Read the model definition and answer for the solid it produces. Units are mm, in the model's axes. Face numbers are marked on the shaded views. A direction names the side the tool comes from. Round coordinates to 2 decimals unless told otherwise and drop trailing zeros. Order: outer loops, then holes, each group sorted by start corner. A loop starts at its lowest first (then second) coordinate and runs counter-clockwise, first axis right, second up. Notation, with made-up numbers: (60.5, 45.5) - (104.5, 45.5) arc R19 ccw to (104.5, 69.5) - close; hole circle Ø4 at (-40, 4). An arc over 180 degrees is marked (long way). Answer as a JSON object with one key per item and string values. Group by question number.
Q1. A cutting plane is placed at A-A on x = 0.5. Determine the outline of the cut face in (y, z).
Q2. Given pin 1 Ø0.5 at (x, z) = (3.5, 0) entering from +Y; pin 2 Ø0.7 at (y, z) = (0, 2) entering from +X, each flat-ended and moving along its own axis, determine where each tip first touches the part or whether it passes through.
Q3. A cutting plane is placed at B-B on y = 0.55. Determine the outline of the cut face in (x, z) (3 decimals), and give its area (3 significant figures).
Q4. A tool of negligible diameter and unlimited length cuts with its end or side. For the marked faces 1 and 2, from which of +Z, -Z, +X, -X, +Y, -Y can it reach the whole face along a straight path? Write none if from no direction.
Q5. Consider line 1 (X direction, y = 0.55, z = 1); line 2 (Z direction, x = -1.5, y = 0.25); line 3 (X direction, y = -0.45, z = 2) (3 decimals). Determine where each line is inside the solid, lowest interval first.
Q6. A cutting plane is placed at D-D on y = -0.8. Determine the outline of the cut face in (x, z), and give its area (3 significant figures).
Q7. A cutting plane is placed at C-C on z = 1.1. Determine the outline of the cut face in (x, y), and give its area (3 significant figures).
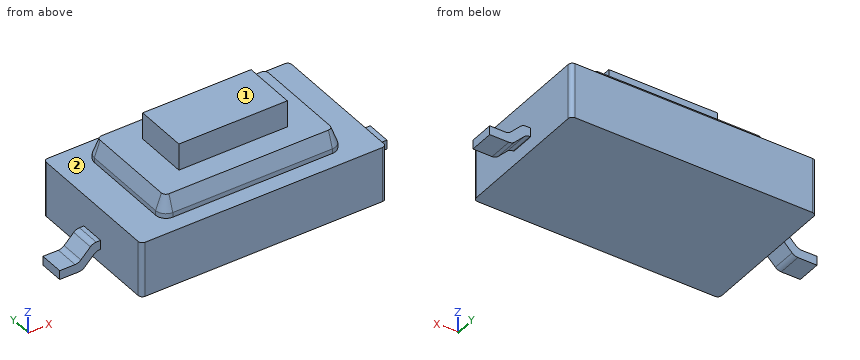
```python
from build123d import *

# Parameters (mm, degrees)
BOSS_EXTRUDE1_DEPTH = 1.35
BOSS_EXTRUDE2_DEPTH = 1.85
SKETCH1_4_W         = 2.65
SKETCH1_4_H         = 1.3
BOSS_EXTRUDE3_DEPTH = 2.5
CHAMFER1_SIZE       = 0.14
CHAMFER1_SIZE2      = 0.384646839
BOSS_EXTRUDE4_DEPTH = 0.3


with BuildPart() as part:
    # Sketch1 → Boss-Extrude1 (new body)
    with BuildSketch(Plane.XY):
        with BuildLine():
            Line((-2.9, 1.75), (2.9, 1.75))
            ThreePointArc((2.9, 1.75), (2.970710678, 1.720710678), (3, 1.65))
            Line((3, 1.65), (3, -1.65))
            ThreePointArc((3, -1.65), (2.970710678, -1.720710678), (2.9, -1.75))
            Line((2.9, -1.75), (-2.9, -1.75))
            ThreePointArc((-2.9, -1.75), (-2.970710678, -1.720710678), (-3, -1.65))
            Line((-3, -1.65), (-3, 1.65))
            ThreePointArc((-3, 1.65), (-2.970710678, 1.720710678), (-2.9, 1.75))
        make_face()
    extrude(amount=BOSS_EXTRUDE1_DEPTH)

    # Sketch1<3> → Boss-Extrude2 (add)
    with BuildSketch(Plane.XY):
        with BuildLine():
            Line((-1.95, 1.35), (1.95, 1.35))
            ThreePointArc((1.95, 1.35), (2.126776695, 1.276776695), (2.2, 1.1))
            Line((2.2, 1.1), (2.2, -1.1))
            ThreePointArc((2.2, -1.1), (2.126776695, -1.276776695), (1.95, -1.35))
            Line((1.95, -1.35), (-1.95, -1.35))
            ThreePointArc((-1.95, -1.35), (-2.126776695, -1.276776695), (-2.2, -1.1))
            Line((-2.2, -1.1), (-2.2, 1.1))
            ThreePointArc((-2.2, 1.1), (-2.126776695, 1.276776695), (-1.95, 1.35))
        make_face()
    extrude(amount=BOSS_EXTRUDE2_DEPTH)

    # Sketch1<4> → Boss-Extrude3 (add)
    with BuildSketch(Plane.XY):
        Rectangle(SKETCH1_4_W, SKETCH1_4_H)
    extrude(amount=BOSS_EXTRUDE3_DEPTH)

    # Chamfer1
    chamfer1_edges = [part.edges().sort_by_distance(p)[0] for p in [
        (0, -1.35, 1.85),
        (-2.126776695, -1.276776695, 1.85),
        (-2.2, 0, 1.85),
        (-2.126776695, 1.276776695, 1.85),
        (2.2, 0, 1.85),
        (2.126776695, 1.276776695, 1.85),
        (0, 1.35, 1.85),
    ]]
    chamfer1_side = [part.faces().sort_by_distance(p)[0] for p in [
        (0, 1.298376362, 1.85),
    ]]
    chamfer(chamfer1_edges, length=CHAMFER1_SIZE, length2=CHAMFER1_SIZE2, reference=chamfer1_side[0])

    # Sketch2 → Boss-Extrude4 (add, symmetric)
    with BuildSketch(Plane(origin=(0, 0, 0), x_dir=(1, 0, 0), z_dir=(0, 1, 0))):
        with BuildLine():
            Line((3, -0.35), (3.017157288, -0.35))
            ThreePointArc((3.017157288, -0.35), (3.093693974, -0.334775907), (3.158578644, -0.291421356))
            Line((3.158578644, -0.291421356), (3.391421356, -0.058578644))
            ThreePointArc((3.391421356, -0.058578644), (3.456306026, -0.015224093), (3.532842712, 0))
            Line((3.532842712, 0), (4, 0))
            Line((4, 0), (4, -0.22))
            Line((4, -0.22), (3.623969696, -0.22))
            ThreePointArc((3.623969696, -0.22), (3.54743301, -0.235224093), (3.48254834, -0.278578644))
            Line((3.48254834, -0.278578644), (3.249705627, -0.511421356))
            ThreePointArc((3.249705627, -0.511421356), (3.184820958, -0.554775907), (3.108284271, -0.57))
            Line((3.108284271, -0.57), (3, -0.57))
            Line((3, -0.57), (3, -0.35))
        make_face()
    boss_extrude4 = extrude(amount=BOSS_EXTRUDE4_DEPTH, both=True)

    # Mirror1: Boss-Extrude4 across plane
    add(boss_extrude4.mirror(Plane(origin=(0, 0, 0), x_dir=(0, 0, 1), z_dir=(1, 0, 0))))


solid = part.part
```
Result set:
{
 "1": {"outline": "(-1.75, 0) - (1.75, 0) - (1.75, 1.35) - (1.35, 1.35) - (1.35, 1.47) - (1.21, 1.85) - (0.65, 1.85) - (0.65, 2.5) - (-0.65, 2.5) - (-0.65, 1.85) - (-1.21, 1.85) - (-1.35, 1.47) - (-1.35, 1.35) - (-1.75, 1.35) - close"},
 "2": {"pin 1": "stops at y = 0.3", "pin 2": "stops at x = 2.13"},
 "3": {"outline": "(-3, 0) - (3, 0) - (3, 1.35) - (2.2, 1.35) - (2.2, 1.465) - (2.06, 1.85) - (1.325, 1.85) - (1.325, 2.5) - (-1.325, 2.5) - (-1.325, 1.85) - (-2.06, 1.85) - (-2.2, 1.465) - (-2.2, 1.35) - (-3, 1.35) - close", "area": "12.0 mm²"},
 "4": {"face 1": "+Z, +X, -X, +Y, -Y", "face 2": "+Z"},
 "5": {"line 1": "x = -3 to 3", "line 2": "z = 0 to 1.85", "line 3": "x = -1.325 to 1.325"},
 "6": {"outline": "(-3, 0) - (3, 0) - (3, 1.35) - (2.2, 1.35) - (2.2, 1.47) - (2.06, 1.85) - (-2.06, 1.85) - (-2.2, 1.47) - (-2.2, 1.35) - (-3, 1.35) - close", "area": "10.2 mm²"},
 "7": {"outline": "(-3, -1.65) arc R0.1 ccw to (-2.9, -1.75) - (2.9, -1.75) arc R0.1 ccw to (3, -1.65) - (3, 1.65) arc R0.1 ccw to (2.9, 1.75) - (-2.9, 1.75) arc R0.1 ccw to (-3, 1.65) - close", "area": "21.0 mm²"}
}
